Source: three-view drawing plus pictorial views. Frame: mm from the lowest corner of the part. Give positions to 0.01 mm unless a question says otherwise; leave off trailing zeros. Loops run counter-clockwise (first coordinate to the right, second up) from the corner with the lowest first, then second, coordinate; pieces in that order, holes last. Notation, with made-up numbers: M 44,61 L 59,61 A21 cw 59,67 Z; hole C 11,42.25 d1. An arc over 180 degrees is marked long. One line per item, written item: value. Start each with the question number.
(1) Section B-B on y = 7.5. Output: boundary loops of the cut face in (x, z).
(2) Pin query (flat end, axial travel): P1, Ø1, axis at x = 68.5, z = 7, coming from the +Y side; P2, Ø2.5, axis at x = 5, z = 5, coming from the -Y side. Return the tip coordinate at first contact, or that it passes through.
(3) Section C-C on x = 85. Output: boundary loops of the cut face in (y, z).
(4) Section A-A on z = 5. Output: boundary loops of the cut face in (x, y).
(5) Ray query, line 1 along X through (y, z) = (5.5, 5); line 2 along X through (y, z) = (9, 5.75); line 3 along Z through (x, y) = (52.5, 4.75). Return the intervals inside material, ascending. Write a range as from..to.
(6) Section D-D on z = 9. Output: boundary loops of the cut face in (x, y), plus the area to 3 significant figures.
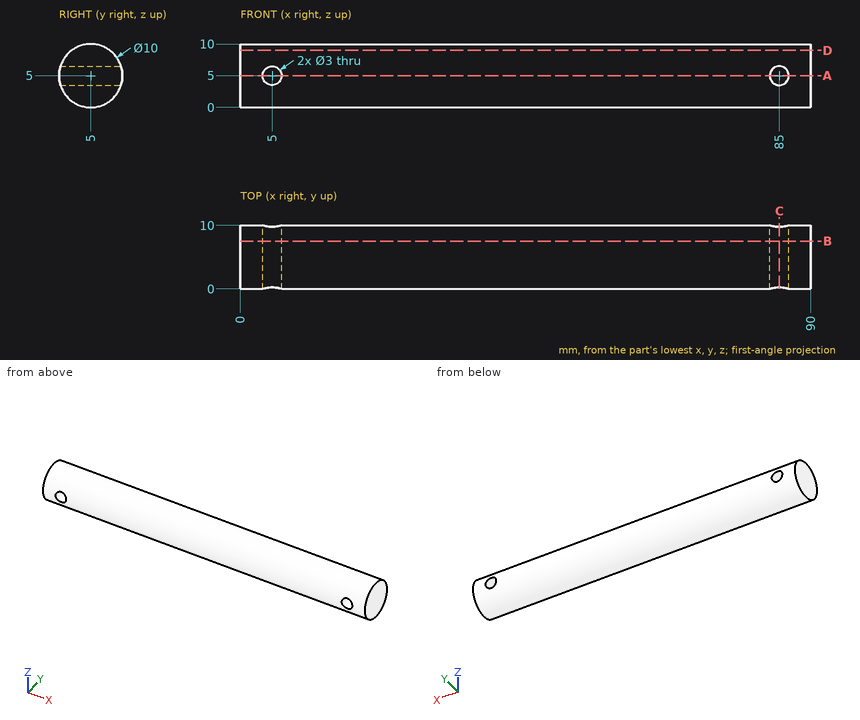
Output values:
1. outline: M 0,0.67 L 90,0.67 L 90,9.33 L 0,9.33 Z; hole C 5,5 d3; hole C 85,5 d3
2. P1: stops at y = 9.77
2. P2: passes through
3. outline: M 0.23,3.5 A5 ccw 9.77,3.5 Z; M 0.23,6.5 L 9.77,6.5 A5 ccw Z
4. outline: M 0,0 L 3.5,0 L 3.5,10 L 0,10 Z; M 6.5,0 L 83.5,0 L 83.5,10 L 6.5,10 Z; M 86.5,0 L 90,0 L 90,10 L 86.5,10 Z
5. line 1: x = 0..3.5, 6.5..83.5, 86.5..90
5. line 2: x = 0..3.7, 6.3..83.7, 86.3..90
5. line 3: z = 0.01..9.99
6. outline: M 0,2 L 90,2 L 90,8 L 0,8 Z
6. area: 540 mm²
